Read the model definition and answer for the solid it produces. Units are mm, in the model's axes. Coordinates: 2 decimals unless noted, no trailing zeros. Loops run counter-clockwise (first coordinate to the right, second up) from the corner with the lowest first, then second, coordinate; pieces in that order, holes last. Notation, with made-up numbers: (73.5, 23) - (109.5, 23) arc R27 cw to (109.5, 50) - close; hole circle Ø1 at (3.25, 42). An arc over 180 degrees is marked (long way). One line per item, written item: value. Start each with the question number.
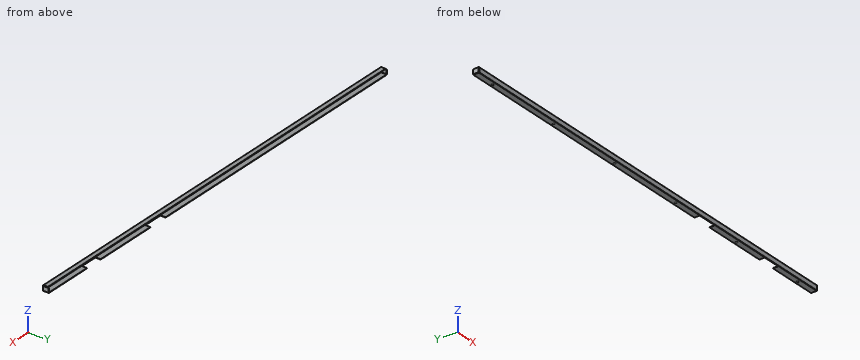
from build123d import *

# Parameters (mm, degrees)
SKETCH_1_W                         = 2104
SKETCH_1_H                         = 21
SM_BASE_FLANGE_1_DEPTH             = 2
SM_EDGE_FLANGE_1_STRIP_W           = 9.4732
SM_EDGE_FLANGE_1_STRIP_H           = 2
SM_EDGE_FLANGE_1_STRIP_CUT_DEPTH   = 2104
SM_EDGE_FLANGE_1_DEPTH             = 2104
SM_EDGE_FLANGE_2_STRIP_W           = 9.4732
SM_EDGE_FLANGE_2_STRIP_H           = 2
SM_EDGE_FLANGE_2_STRIP_CUT_DEPTH   = 2104
SM_EDGE_FLANGE_2_DEPTH             = 2104
SM_EDGE_FLANGE_3_STRIP_W           = 9.4732
SM_EDGE_FLANGE_3_STRIP_H           = 2
SM_EDGE_FLANGE_3_STRIP_CUT_DEPTH   = 25.2634
SM_EDGE_FLANGE_3_STRIP_2_W         = 9.4732
SM_EDGE_FLANGE_3_STRIP_2_H         = 2
SM_EDGE_FLANGE_3_STRIP_CUT_2_DEPTH = 25.2634
SM_EDGE_FLANGE_3_DEPTH             = 25.2634
SM_EDGE_FLANGE_3_BEND_DEPTH        = 25.2634
SKETCH_18_W                        = 85
SKETCH_18_H                        = 39.234140159
SKETCH_18_W_2                      = 95
SKETCH_18_H_2                      = 42.308601705
CUT_EXTRUDE_1_DEPTH                = 2
SKETCH_19_R                        = 6
CUT_EXTRUDE_2_DEPTH                = 0.1


# Sheet-metal steps are written as plain solids
with BuildPart() as part:
    # Sketch 1 → 基体-法兰1 (new body)
    with BuildSketch(Plane.XY):
        with Locations((-1050, 7.5)):
            Rectangle(SKETCH_1_W, SKETCH_1_H)
    extrude(amount=SM_BASE_FLANGE_1_DEPTH)

    # 边线-法兰1 strip (across the edge) → 边线-法兰1 strip cut (cut)
    with BuildSketch(Plane(origin=(2, -3, 0), x_dir=(0, 1, 0), z_dir=(-1, 0, 0))):
        with Locations((-4, -1)):
            Rectangle(SM_EDGE_FLANGE_1_STRIP_W, SM_EDGE_FLANGE_1_STRIP_H)
    extrude(amount=SM_EDGE_FLANGE_1_STRIP_CUT_DEPTH, mode=Mode.SUBTRACT)

    # 边线-法兰1 section (across the edge) → 边线-法兰1 (add)
    with BuildSketch(Plane(origin=(2, -3, 0), x_dir=(0, 1, 0), z_dir=(-1, 0, 0))):
        with BuildLine():
            Line((-2, 0.7366), (-2, 21))
            Line((-2, 21), (0, 21))
            Line((0, 21), (0, 0.7366))
            ThreePointArc((0, 0.7366), (0.215745145, 0.215745145), (0.7366, 0))
            Line((0.7366, 0), (0.7366, -2))
            ThreePointArc((0.7366, -2), (-1.198468417, -1.198468417), (-2, 0.7366))
        make_face()
    extrude(amount=SM_EDGE_FLANGE_1_DEPTH)

    # 边线-法兰2 strip (across the edge) → 边线-法兰2 strip cut (cut)
    with BuildSketch(Plane(origin=(2, -3, -21), x_dir=(0, 0, 1), z_dir=(-1, 0, 0))):
        with Locations((-4, -1)):
            Rectangle(SM_EDGE_FLANGE_2_STRIP_W, SM_EDGE_FLANGE_2_STRIP_H)
    extrude(amount=SM_EDGE_FLANGE_2_STRIP_CUT_DEPTH, mode=Mode.SUBTRACT)

    # 边线-法兰2 section (across the edge) → 边线-法兰2 (add)
    with BuildSketch(Plane(origin=(2, -3, -21), x_dir=(0, 0, 1), z_dir=(-1, 0, 0))):
        with BuildLine():
            Line((-2, 0.7366), (-2, 26))
            Line((-2, 26), (0, 26))
            Line((0, 26), (0, 0.7366))
            ThreePointArc((0, 0.7366), (0.215745145, 0.215745145), (0.7366, 0))
            Line((0.7366, 0), (0.7366, -2))
            ThreePointArc((0.7366, -2), (-1.198468417, -1.198468417), (-2, 0.7366))
        make_face()
    extrude(amount=SM_EDGE_FLANGE_2_DEPTH)

    # 边线-法兰3 strip (across the edge) → 边线-法兰3 strip cut (cut)
    with BuildSketch(Plane(origin=(2, -2.2634, -21), x_dir=(-1, 0, 0), z_dir=(0, 1, 0))):
        with Locations((-4, -1)):
            Rectangle(SM_EDGE_FLANGE_3_STRIP_W, SM_EDGE_FLANGE_3_STRIP_H)
    extrude(amount=SM_EDGE_FLANGE_3_STRIP_CUT_DEPTH, mode=Mode.SUBTRACT)

    # 边线-法兰3 strip 2 (across the edge) → 边线-法兰3 strip cut 2 (cut)
    with BuildSketch(Plane(origin=(-2102, 23, -21), x_dir=(1, 0, 0), z_dir=(0, -1, 0))):
        with Locations((-4, -1)):
            Rectangle(SM_EDGE_FLANGE_3_STRIP_2_W, SM_EDGE_FLANGE_3_STRIP_2_H)
    extrude(amount=SM_EDGE_FLANGE_3_STRIP_CUT_2_DEPTH, mode=Mode.SUBTRACT)

    # 边线-法兰3 section (across the edge) → 边线-法兰3 (add)
    with BuildSketch(Plane(origin=(2, -2.2634, -21), x_dir=(-1, 0, 0), z_dir=(0, 1, 0))):
        with BuildLine():
            Line((-2, 0.7366), (-2, 20))
            Line((-2, 20), (0, 20))
            Line((0, 20), (0, 0.7366))
            ThreePointArc((0, 0.7366), (0.215745145, 0.215745145), (0.7366, 0))
            Line((0.7366, 0), (0.7366, -2))
            ThreePointArc((0.7366, -2), (-1.198468417, -1.198468417), (-2, 0.7366))
        make_face()
    extrude(amount=SM_EDGE_FLANGE_3_DEPTH)

    # 边线-法兰3 section 2 (across the edge) → 边线-法兰3 bend (add)
    with BuildSketch(Plane(origin=(-2102, 23, -21), x_dir=(1, 0, 0), z_dir=(0, -1, 0))):
        with BuildLine():
            Line((-2, 0.7366), (-2, 20))
            Line((-2, 20), (0, 20))
            Line((0, 20), (0, 0.7366))
            ThreePointArc((0, 0.7366), (0.215745145, 0.215745145), (0.7366, 0))
            Line((0.7366, 0), (0.7366, -2))
            ThreePointArc((0.7366, -2), (-1.198468417, -1.198468417), (-2, 0.7366))
        make_face()
    extrude(amount=SM_EDGE_FLANGE_3_BEND_DEPTH)

    # 草图18 → 切除-拉伸1 (cut)
    with BuildSketch(Plane(origin=(0, 0, -23), x_dir=(-1, 0, 0), z_dir=(0, 0, -1))):
        with Locations((277.5, 17.35367008)):
            Rectangle(SKETCH_18_W, SKETCH_18_H)
        with Locations((677.5, 18.890900853)):
            Rectangle(SKETCH_18_W_2, SKETCH_18_H_2)
    extrude(amount=-CUT_EXTRUDE_1_DEPTH, mode=Mode.SUBTRACT)

    # 草图19 → 切除-拉伸2 (cut)
    with BuildSketch(Plane(origin=(0, 0, -23), x_dir=(-1, 0, 0), z_dir=(0, 0, -1))):
        with Locations((98.7366, 10.3683)):
            Circle(SKETCH_19_R)
        with Locations((478.7366, 10.3683)):
            Circle(SKETCH_19_R)
        with Locations((858.7366, 10.3683)):
            Circle(SKETCH_19_R)
        with Locations((1238.7366, 10.3683)):
            Circle(SKETCH_19_R)
        with Locations((1618.7366, 10.3683)):
            Circle(SKETCH_19_R)
        with Locations((1998.7366, 10.3683)):
            Circle(SKETCH_19_R)
    extrude(amount=-CUT_EXTRUDE_2_DEPTH, mode=Mode.SUBTRACT)


solid = part.part
1) Section B-B, the plane x = -1463 is taken. Determine the outline of the cut face in (y, z).
2) Straight lines are drawn through the part: L1, parallel to X at y = 14.75, z = -16.5; L2, parallel to Z at x = -806.5, y = 1.75; L3, parallel to X at y = 16, z = -20.75. For each, find the intervals that lie inside material, in ascending order.
3) Section C-C, the plane x = -688 is taken. Determine the outline of the cut face in (y, z).
4) Section A-A, the plane z = -16 is taken. Determine the outline of the cut face in (x, y).
5) Flat-ended cylindrical pins translate along their axes: P1, Ø1, axis at y = 12.5, z = -22, coming from the -X side; P2, Ø1, axis at y = 11, z = -21.5, coming from the +X side; P3, Ø0.6, axis at x = -2102.5, y = 7, coming from the +Z side. Find the tip coordinate at first contact, or state that the pin passes through.
Answer below:
1. outline: (-5, -20.26) arc R2.74 ccw to (-2.26, -23) - (23, -23) - (23, -21) - (-2.26, -21) arc R0.74 cw to (-3, -20.26) - (-3, -0.74) arc R0.74 cw to (-2.26, 0) - (18, 0) - (18, 2) - (-2.26, 2) arc R2.74 ccw to (-5, -0.74) - close
2. L1: -2104 to -2102, 2 to 4
2. L2: -23 to -21, 0 to 2
2. L3: -2103.96 to -2101.82, 1.82 to 3.96
3. outline: (-5, -20.26) arc R2.74 ccw to (-2.26, -23) - (-2.26, -21) arc R0.74 cw to (-3, -20.26) - (-3, -0.74) arc R0.74 cw to (-2.26, 0) - (18, 0) - (18, 2) - (-2.26, 2) arc R2.74 ccw to (-5, -0.74) - close
4. outline: (-2104, -2.26) - (-2102, -2.26) - (-2102, 23) - (-2104, 23) - close; (-2102, -5) - (2, -5) - (2, -3) - (-2102, -3) - close; (2, -2.26) - (4, -2.26) - (4, 23) - (2, 23) - close
5. P1: x = -2103.7
5. P2: x = 3.9
5. P3: z = -1
